Source: CAD feature listing. Evaluate the final solid. Frame: model axes, mm. A direction names the side the tool comes from. Give positions to 0.01 mm unless a question says otherwise; leave off trailing zeros. Loops run counter-clockwise (first coordinate to the right, second up) from the corner with the lowest first, then second, coordinate; pieces in that order, holes last. Notation, with made-up numbers: M 81,-1.5 L 133,-1.5 A35 cw 133,35.5 Z; hole C 2,-31.5 d6. An arc over 180 degrees is marked long. Put each result on its own line as item: value.
from build123d import *

# Parameters (mm, degrees)
PAD_DEPTH    = 8
THICKNESS_T  = -1
POCKET_DEPTH = 0.5
PAD001_DEPTH = 8
PAD002_DEPTH = 8
SKETCH003_W  = 1
SKETCH003_H  = 7.5
PAD003_DEPTH = 18
SKETCH004_W  = 1
SKETCH004_H  = 7.5
PAD004_DEPTH = 18
SKETCH005_W  = 1
SKETCH005_H  = 7.5
PAD005_DEPTH = 18
SKETCH006_W  = 1
SKETCH006_H  = 7.5
PAD006_DEPTH = 18
SKETCH007_W  = 1
SKETCH007_H  = 7.5
PAD007_DEPTH = 7
SKETCH008_W  = 1
SKETCH008_H  = 7.5
PAD008_DEPTH = 7
SKETCH009_W  = 1
SKETCH009_H  = 7.5
PAD009_DEPTH = 7
SKETCH010_W  = 1
SKETCH010_H  = 7.5
PAD010_DEPTH = 7


with BuildPart() as part:
    # Sketch → Pad (new body)
    with BuildSketch(Plane.XY):
        Polygon((-29.21, 38.1002724549), (-29.21, -38.0997275451), (-13.9697275451, -53.34), (13.9702724549, -53.34), (29.2105449098, -38.0997275451), (29.2105449098, 38.1002724549), (13.9702724549, 53.3405449098), (-13.9697275451, 53.3405449098), align=None)
        Polygon((-19.05, 35.5607622358), (-19.05, 12.7007622358), (-11.4302173259, 5.0809795617), (11.4297826741, 5.0809795617), (19.0495653481, 12.7007622358), (19.0495653481, 35.5607622358), (11.4297826741, 43.1805449098), (-11.4302173259, 43.1805449098), align=None, mode=Mode.SUBTRACT)
        Polygon((-19.05, -35.5602173259), (-19.05, -12.7002173259), (-11.4302173259, -5.0804346519), (11.4297826741, -5.0804346519), (19.0495653481, -12.7002173259), (19.0495653481, -35.5602173259), (11.4297826741, -43.18), (-11.4302173259, -43.18), align=None, mode=Mode.SUBTRACT)
    extrude(amount=PAD_DEPTH)

    # Thickness
    thickness_openings = [part.faces().sort_by_distance(p)[0] for p in [
        (0.000695, 0.000272, 8),
    ]]
    offset(amount=THICKNESS_T, openings=thickness_openings, kind=Kind.INTERSECTION)

    # Thickness Face35 → Pocket (cut)
    with BuildSketch(Plane(origin=(0.0008428897, 0.0002724549, 1), x_dir=(0, 1, 0), z_dir=(0, 0, 1))):
        Polygon((37.6857864376, 28.2108428897), (-37.6857864376, 28.2108428897), (-52.3402724549, 13.5563568724), (-52.3402724549, -13.5552160028), (-37.6857864376, -28.2097020201), (37.6857864376, -28.2097020201), (52.3402724549, -13.5552160028), (52.3402724549, 13.5563568724), align=None)
        Polygon((35.9747033432, 20.0508428897), (44.1802724549, 11.845273778), (44.1802724549, -11.8431533467), (35.9747033432, -20.0487224584), (12.2862762185, -20.0487224584), (4.0807071068, -11.8431533467), (4.0807071068, 11.845273778), (12.2862762185, 20.0508428897), align=None, mode=Mode.SUBTRACT)
        Polygon((-35.9747033432, 20.0508428897), (-12.2862762185, 20.0508428897), (-4.0807071068, 11.845273778), (-4.0807071068, -11.8431533467), (-12.2862762185, -20.0487224584), (-35.9747033432, -20.0487224584), (-44.1802724549, -11.8431533467), (-44.1802724549, 11.845273778), align=None, mode=Mode.SUBTRACT)
    extrude(amount=-POCKET_DEPTH, mode=Mode.SUBTRACT)

    # Sketch001 → Pad001 (join)
    with BuildSketch(Plane.XZ.offset(35.56)):
        Polygon((-19.05, 4), (-19.05, 9.8), (-19.85, 9.8), (-19.85, 11), (-17.05, 11), (-17.05, 7), align=None)
        Polygon((19.05, 4), (19.05, 9.8), (19.85, 9.8), (19.85, 11), (17.05, 11), (17.05, 7), align=None)
    extrude(amount=-PAD001_DEPTH)

    # Sketch002 → Pad002 (join)
    with BuildSketch(Plane.XZ.offset(-35.56)):
        Polygon((-19.05, 4), (-19.05, 9.8), (-19.85, 9.8), (-19.85, 11), (-17.05, 11), (-17.05, 7), align=None)
        Polygon((19.05, 4), (19.05, 9.8), (19.85, 9.8), (19.85, 11), (17.05, 11), (17.05, 7), align=None)
    extrude(amount=PAD002_DEPTH)

    # Sketch003 (on Face77 of Pad002) → Pad003 (join)
    with BuildSketch(Plane(origin=(3.8815083374, -3.8815083374, 0), x_dir=(0.7071067812, 0.7071067812, 0), z_dir=(0.7071067812, -0.7071067812, 0))):
        with Locations((17.0628719395, 4.25)):
            Rectangle(SKETCH003_W, SKETCH003_H)
    extrude(amount=PAD003_DEPTH)

    # Sketch004 (on Face56 of Pad003) → Pad004 (join)
    with BuildSketch(Plane(origin=(3.8817807923, 3.8817807923, 0), x_dir=(-0.7071067812, 0.7071067812, 0), z_dir=(0.7071067812, 0.7071067812, 0))):
        with Locations((-17.06248663, 4.25)):
            Rectangle(SKETCH004_W, SKETCH004_H)
    extrude(amount=PAD004_DEPTH)

    # Sketch005 (on Face84 of Pad004) → Pad005 (join)
    with BuildSketch(Plane(origin=(-3.8817256633, -3.8817256633, 0), x_dir=(0.7071067812, -0.7071067812, 0), z_dir=(-0.7071067812, -0.7071067812, 0))):
        with Locations((-17.0631792847, 4.25)):
            Rectangle(SKETCH005_W, SKETCH005_H)
    extrude(amount=PAD005_DEPTH)

    # Sketch006 (on Face69 of Pad005) → Pad006 (join)
    with BuildSketch(Plane(origin=(-3.8819981182, 3.8819981182, 0), x_dir=(-0.7071067812, -0.7071067812, 0), z_dir=(-0.7071067812, 0.7071067812, 0))):
        with Locations((17.0627939753, 4.25)):
            Rectangle(SKETCH006_W, SKETCH006_H)
    extrude(amount=PAD006_DEPTH)

    # Sketch007 (on Face79 of Pad006) → Pad007 (join)
    with BuildSketch(Plane(origin=(-28.0124878991, 28.0124878991, 0), x_dir=(-0.7071067812, -0.7071067812, 0), z_dir=(-0.7071067812, 0.7071067812, 0))):
        with Locations((-17.0628719395, 4.25)):
            Rectangle(SKETCH007_W, SKETCH007_H)
    extrude(amount=PAD007_DEPTH)

    # Sketch008 (on Face73 of Pad007) → Pad008 (join)
    with BuildSketch(Plane(origin=(-28.0122154442, -28.0122154442, 0), x_dir=(0.7071067812, -0.7071067812, 0), z_dir=(-0.7071067812, -0.7071067812, 0))):
        with Locations((17.06248663, 4.25)):
            Rectangle(SKETCH008_W, SKETCH008_H)
    extrude(amount=PAD008_DEPTH)

    # Sketch009 (on Face64 of Pad008) → Pad009 (join)
    with BuildSketch(Plane(origin=(28.0119981182, -28.0119981182, 0), x_dir=(0.7071067812, 0.7071067812, 0), z_dir=(0.7071067812, -0.7071067812, 0))):
        with Locations((-17.0627939753, 4.25)):
            Rectangle(SKETCH009_W, SKETCH009_H)
    extrude(amount=PAD009_DEPTH)

    # Sketch010 (on Face62 of Pad009) → Pad010 (join)
    with BuildSketch(Plane(origin=(28.0122705731, 28.0122705731, 0), x_dir=(-0.7071067812, 0.7071067812, 0), z_dir=(0.7071067812, 0.7071067812, 0))):
        with Locations((17.0631792847, 4.25)):
            Rectangle(SKETCH010_W, SKETCH010_H)
    extrude(amount=PAD010_DEPTH)


solid = part.part
1. Section query A-A (y = 29.5). Output: boundary loops of the cut face in (x, z), plus the area to 3 significant figures.
Found:
outline: M -29.21,0 L -19.05,0 L -19.05,4 L -17.05,7 L -17.05,11 L -19.85,11 L -19.85,9.8 L -19.05,9.8 L -19.05,8 L -20.05,8 L -20.05,0.5 L -28.21,0.5 L -28.21,8 L -29.21,8 Z; M 17.05,7 L 19.05,4 L 19.05,0 L 29.21,0 L 29.21,8 L 28.21,8 L 28.21,0.5 L 20.05,0.5 L 20.05,8 L 19.05,8 L 19.05,9.8 L 19.85,9.8 L 19.85,11 L 17.05,11 Z
area: 64.1 mm^2
2. Material intervals for line 1 (X direction, y = 26.5, z = 4); line 2 (Y direction, x = 8, z = 5.5); line 3 (X direction, y = -42.5, z = 1), sorted ascending. Write a range as from..to.
Found:
line 1: -29.21..-28.21, -20.05..-19.05, 19.05..20.05, 28.21..29.21
line 2: -53.34..-52.34, -44.18..-43.18, -5.08..-4.08, 4.08..5.08, 43.18..44.18, 52.34..53.34
line 3: -24.81..-23.4, -19.08..-17.66, -13.52..-12.11, 12.11..13.52, 17.66..19.08, 23.4..24.81
3. Access query for faces 1 (the flat face through (0, -5.08, 4)), 2 (the flat face through (19.05, -21, 4)), 3 (the flat face through (18, -27.56, 8)). Directions: +Z, -Z, +X, -X, +Y, -Y. A direction counts if a zero-diameter tool reaches every point of the face in a straight line with its end or side. Return the directions, or none.
Found:
face 1: +Z, -Z
face 2: -Z
face 3: +Z
4. Section query D-D (y = 6.5). Output: boundary loops of the cut face in (x, z).
Found:
outline: M -29.21,0 L -12.85,0 L -12.85,8 L -14.26,8 L -14.26,0.5 L -16.92,0.5 L -16.92,8 L -18.34,8 L -18.34,0.5 L -28.21,0.5 L -28.21,8 L -29.21,8 Z; M 12.85,0 L 29.21,0 L 29.21,8 L 28.21,8 L 28.21,0.5 L 18.34,0.5 L 18.34,8 L 16.92,8 L 16.92,0.5 L 14.26,0.5 L 14.26,8 L 12.85,8 Z
5. Section query B-B (x = 5.5). Output: boundary loops of the cut face in (y, z).
Found:
outline: M -53.34,0 L -43.18,0 L -43.18,8 L -44.18,8 L -44.18,0.5 L -52.34,0.5 L -52.34,8 L -53.34,8 Z; M -5.08,0 L 5.08,0 L 5.08,8 L 4.08,8 L 4.08,0.5 L -4.08,0.5 L -4.08,8 L -5.08,8 Z; M 43.18,0 L 53.34,0 L 53.34,8 L 52.34,8 L 52.34,0.5 L 44.18,0.5 L 44.18,8 L 43.18,8 Z
6. Contact query for flat-ended pins moving along their axis: P1, Ø3, axis at x = 22, z = 8, coming from the -Y side; P2, Ø3, axis at x = 18.5, z = 8, coming from the +Y side; P3, Ø9.5, axis at x = -3.5, y = 46, coming from the +Z side. Output: stop coordinate, or through.
Found:
P1: y = -46.81
P2: y = 50.31
P3: z = 8
7. Section query C-C (z = 2.5). State how many separate pieces and enclosed holes the cut face has, plus the area to 3 significant figures.
Found:
separate pieces: 1
enclosed holes: 11
area: 662 mm^2
